Source: CAD feature listing. Evaluate the final solid. Frame: model axes, mm. A direction names the side the tool comes from. Give positions to 0.01 mm unless a question says otherwise; leave off trailing zeros. Loops run counter-clockwise (first coordinate to the right, second up) from the corner with the lowest first, then second, coordinate; pieces in that order, holes last.
from build123d import *
from build123d.topology import SkipClean

# Parameters (mm, degrees)
BOSS_EXTRU_1_DEPTH      = 20
COQUE1_START            = -48.5
COQUE1_OUTLINE_W        = 78
COQUE1_OUTLINE_H        = 18
COQUE1_DEPTH            = 97
ENL_V_MAT_EXTRU_1_DEPTH = 99.357765326
ESQUISSE3_W             = 3
ESQUISSE3_H             = 5
ESQUISSE3_W_2           = 6
ESQUISSE3_H_2           = 3
BOSS_EXTRU_2_DEPTH      = 8
ESQUISSE4_W             = 1.5
ESQUISSE4_H             = 2
ENL_V_MAT_EXTRU_2_DEPTH = 5
CHANFREIN1_SIZE         = 2
ESQUISSE5_W             = 2
ESQUISSE5_H             = 2
ENL_V_MAT_EXTRU_3_DEPTH = 6
CHANFREIN2_SIZE         = 2
ESQUISSE7_W             = 8
ESQUISSE7_H             = 3
ENL_V_MAT_EXTRU_4_DEPTH = 6
CHANFREIN3_SIZE         = 1
ESQUISSE9_R             = 1
ENL_V_MAT_EXTRU_5_DEPTH = 68.492592186
ESQUISSE10_R            = 1
BOSS_EXTRU_5_DEPTH      = 20
ENL_V_MAT_EXTRU_6_DEPTH = 82


# Read off the part's stored shape, not the designer's step: Coque1
with BuildPart() as part:
    # Esquisse1 → Boss.-Extru.1 (new body)
    with BuildSketch(Plane.XY):
        with BuildLine():
            Line((-39, 50.5), (39, 50.5))
            ThreePointArc((39, 50.5), (40.414213562, 49.914213562), (41, 48.5))
            Line((41, 48.5), (41, -48.5))
            ThreePointArc((41, -48.5), (40.414213562, -49.914213562), (39, -50.5))
            Line((39, -50.5), (-39, -50.5))
            ThreePointArc((-39, -50.5), (-40.414213562, -49.914213562), (-41, -48.5))
            Line((-41, -48.5), (-41, 48.5))
            ThreePointArc((-41, 48.5), (-40.414213562, 49.914213562), (-39, 50.5))
        make_face()
    extrude(amount=BOSS_EXTRU_1_DEPTH)

    # Coque1 outline → Coque1 (cut)
    with BuildSketch(Plane(origin=(0, 0, 0), x_dir=(1, 0, 0), z_dir=(0, 1, 0)).offset(COQUE1_START)):
        with Locations((0, -11)):
            Rectangle(COQUE1_OUTLINE_W, COQUE1_OUTLINE_H)
    extrude(amount=COQUE1_DEPTH, mode=Mode.SUBTRACT)

    # Esquisse2 → Enlèv. mat.-Extru.1 (cut, through all)
    with BuildSketch(Plane.ZY.offset(41)):
        Polygon((20, -50.5), (15, -50.5), (20, 50.5), align=None)
    extrude(amount=-ENL_V_MAT_EXTRU_1_DEPTH, mode=Mode.SUBTRACT)

    # Esquisse3 → Boss.-Extru.2 (add)
    with BuildSketch(Plane.XY.offset(2)):
        with Locations((10.5, 40.982596477)):
            Rectangle(ESQUISSE3_W, ESQUISSE3_H)
        with Locations((-10.5, 40.982596477)):
            Rectangle(ESQUISSE3_W, ESQUISSE3_H)
        with Locations((0, 15.010755302)):
            Rectangle(ESQUISSE3_W_2, ESQUISSE3_H_2)
    extrude(amount=BOSS_EXTRU_2_DEPTH)

    # Esquisse4 → Enlèv. mat.-Extru.2 (cut)
    with BuildSketch(Plane.XZ.offset(-38.482596477)):
        with Locations((9.75, 7)):
            Rectangle(ESQUISSE4_W, ESQUISSE4_H)
        with Locations((-9.75, 7)):
            Rectangle(ESQUISSE4_W, ESQUISSE4_H)
    extrude(amount=-ENL_V_MAT_EXTRU_2_DEPTH, mode=Mode.SUBTRACT)

    # Chanfrein1
    chanfrein1_edges = [part.edges().sort_by_distance(p)[0] for p in [
        (9, 40.982596477, 10),
        (-9, 40.982596477, 10),
    ]]
    chamfer(chanfrein1_edges, length=CHANFREIN1_SIZE - 0.0001)  # a hair under: the kernel refuses the full size

    # Esquisse5 → Enlèv. mat.-Extru.3 (cut)
    with BuildSketch(Plane.ZY.offset(3)):
        with Locations((7, 15.510755302)):
            Rectangle(ESQUISSE5_W, ESQUISSE5_H)
    extrude(amount=-ENL_V_MAT_EXTRU_3_DEPTH, mode=Mode.SUBTRACT)

    # Chanfrein2
    chanfrein2_edges = [part.edges().sort_by_distance(p)[0] for p in [
        (0, 16.510755302, 10),
    ]]
    chamfer(chanfrein2_edges, length=CHANFREIN2_SIZE - 0.0001)  # a hair under: the kernel refuses the full size

    # Esquisse7 → Enlèv. mat.-Extru.4 (cut)
    with BuildSketch(Plane(origin=(0, 50.5, 0), x_dir=(1, 0, 0), z_dir=(0, 1, 0))):
        with Locations((0, -8.5)):
            Rectangle(ESQUISSE7_W, ESQUISSE7_H)
    extrude(amount=-ENL_V_MAT_EXTRU_4_DEPTH, mode=Mode.SUBTRACT)

    # Chanfrein3
    chanfrein3_edges = [part.edges().sort_by_distance(p)[0] for p in [
        (4, 49.5, 7),
        (-4, 49.5, 7),
    ]]
    chamfer(chanfrein3_edges, length=CHANFREIN3_SIZE)

    # Esquisse9 → Enlèv. mat.-Extru.5 (cut, through all)
    with BuildSketch(Plane.XY.offset(2)):
        with Locations((-39, 48.5)):
            Circle(ESQUISSE9_R)
        with Locations((-39, -48.5)):
            Circle(ESQUISSE9_R)
        with Locations((-39, 0)):
            Circle(ESQUISSE9_R)
        with Locations((39, 0)):
            Circle(ESQUISSE9_R)
        with Locations((39, -48.5)):
            Circle(ESQUISSE9_R)
        with Locations((39, 48.5)):
            Circle(ESQUISSE9_R)
    extrude(amount=ENL_V_MAT_EXTRU_5_DEPTH, mode=Mode.SUBTRACT)

    # Esquisse10 → Boss.-Extru.5 (add)
    # profile 1 of 12: a face of its own
    with SkipClean():  # the faces are left unmerged after this step: merging them gives an invalid solid
        with BuildSketch(Plane.XY):
            with BuildLine():
                Line((-41, 48.5), (-41, 47))
                ThreePointArc((-41, 47), (-38.209430585, 46.128291755), (-36.5, 48.5))
                ThreePointArc((-36.5, 48.5), (-36.763932023, 49.618033989), (-37.5, 50.5))
                Line((-37.5, 50.5), (-39, 50.5))
                ThreePointArc((-39, 50.5), (-40.414213562, 49.914213562), (-41, 48.5))
            make_face()
            with Locations((-39, 48.5)):
                Circle(ESQUISSE10_R, mode=Mode.SUBTRACT)
        # profile 2 of 12: a face of its own
        with BuildSketch(Plane.XY):
            with BuildLine():
                Line((39, 50.5), (37.5, 50.5))
                ThreePointArc((37.5, 50.5), (37.232233047, 46.732233047), (41, 47))
                Line((41, 47), (41, 48.5))
                ThreePointArc((41, 48.5), (40.414213562, 49.914213562), (39, 50.5))
            make_face()
            with Locations(Location((39, 48.5, 0), (0, 0, 180))):
                Circle(ESQUISSE10_R, mode=Mode.SUBTRACT)
        # profile 3 of 12: a face of its own
        with BuildSketch(Plane.XY):
            with BuildLine():
                ThreePointArc((-40, 0), (-39, 1), (-38, 0))
                Line((-38, 0), (-36.5, 0))
                ThreePointArc((-36.5, 0), (-38.209430585, 2.371708245), (-41, 1.5))
                Line((-41, 1.5), (-41, 0))
                Line((-41, 0), (-40, 0))
            make_face()
        # profile 4 of 12: a face of its own
        with BuildSketch(Plane.XY):
            with BuildLine():
                Line((-36.5, 0), (-38, 0))
                ThreePointArc((-38, 0), (-39, -1), (-40, 0))
                Line((-40, 0), (-41, 0))
                Line((-41, 0), (-41, -1.5))
                ThreePointArc((-41, -1.5), (-38.209430585, -2.371708245), (-36.5, 0))
            make_face()
        # profile 5 of 12: a face of its own
        with BuildSketch(Plane.XY):
            with BuildLine():
                ThreePointArc((-40, 0), (-39, 1), (-38, 0))
                Line((-38, 0), (-36.5, 0))
                ThreePointArc((-36.5, 0), (-38.209430585, 2.371708245), (-41, 1.5))
                Line((-41, 1.5), (-41, 0))
                Line((-41, 0), (-40, 0))
            make_face()
        # profile 6 of 12: a face of its own
        with BuildSketch(Plane.XY):
            with BuildLine():
                Line((-36.5, 0), (-38, 0))
                ThreePointArc((-38, 0), (-39, -1), (-40, 0))
                Line((-40, 0), (-41, 0))
                Line((-41, 0), (-41, -1.5))
                ThreePointArc((-41, -1.5), (-38.209430585, -2.371708245), (-36.5, 0))
            make_face()
        # profile 7 of 12: a face of its own
        with BuildSketch(Plane.XY):
            with BuildLine():
                ThreePointArc((-36.5, -48.5), (-38.209430585, -46.128291755), (-41, -47))
                Line((-41, -47), (-41, -48.5))
                ThreePointArc((-41, -48.5), (-40.414213562, -49.914213562), (-39, -50.5))
                Line((-39, -50.5), (-37.5, -50.5))
                ThreePointArc((-37.5, -50.5), (-36.763932023, -49.618033989), (-36.5, -48.5))
            make_face()
            with Locations(Location((-39, -48.5, 0), (0, 0, 180))):
                Circle(ESQUISSE10_R, mode=Mode.SUBTRACT)
        # profile 8 of 12: a face of its own
        with BuildSketch(Plane.XY):
            with BuildLine():
                ThreePointArc((41, -47), (37.232233047, -46.732233047), (37.5, -50.5))
                Line((37.5, -50.5), (39, -50.5))
                ThreePointArc((39, -50.5), (40.414213562, -49.914213562), (41, -48.5))
                Line((41, -48.5), (41, -47))
            make_face()
            with Locations((39, -48.5)):
                Circle(ESQUISSE10_R, mode=Mode.SUBTRACT)
        # profile 9 of 12: a face of its own
        with BuildSketch(Plane.XY):
            with BuildLine():
                ThreePointArc((41, 1.5), (38.209430585, 2.371708245), (36.5, 0))
                Line((36.5, 0), (38, 0))
                ThreePointArc((38, 0), (39, 1), (40, 0))
                Line((40, 0), (41, 0))
                Line((41, 0), (41, 1.5))
            make_face()
        # profile 10 of 12: a face of its own
        with BuildSketch(Plane.XY):
            with BuildLine():
                Line((38, 0), (36.5, 0))
                ThreePointArc((36.5, 0), (38.209430585, -2.371708245), (41, -1.5))
                Line((41, -1.5), (41, 0))
                Line((41, 0), (40, 0))
                ThreePointArc((40, 0), (39, -1), (38, 0))
            make_face()
        # profile 11 of 12: a face of its own
        with BuildSketch(Plane.XY):
            with BuildLine():
                ThreePointArc((41, 1.5), (38.209430585, 2.371708245), (36.5, 0))
                Line((36.5, 0), (38, 0))
                ThreePointArc((38, 0), (39, 1), (40, 0))
                Line((40, 0), (41, 0))
                Line((41, 0), (41, 1.5))
            make_face()
        # profile 12 of 12: a face of its own
        with BuildSketch(Plane.XY):
            with BuildLine():
                Line((38, 0), (36.5, 0))
                ThreePointArc((36.5, 0), (38.209430585, -2.371708245), (41, -1.5))
                Line((41, -1.5), (41, 0))
                Line((41, 0), (40, 0))
                ThreePointArc((40, 0), (39, -1), (38, 0))
            make_face()
        extrude(amount=BOSS_EXTRU_5_DEPTH)
    add(part.part.scale(1), mode=Mode.REPLACE)  # the faces are merged on a copy

    # Esquisse11 → Enlèv. mat.-Extru.6 (cut)
    with BuildSketch(Plane(origin=(-41, 0, -41), x_dir=(0, 0, 1), z_dir=(-1, 0, 0))):
        Polygon((61, -50.68921089), (56, -50.68921089), (61, 50.5), align=None)
    extrude(amount=-ENL_V_MAT_EXTRU_6_DEPTH, mode=Mode.SUBTRACT)


solid = part.part
1) Contact query for flat-ended pins moving along their axis: P1, Ø2.5, axis at x = 39, y = -48.5, coming from the +Z side; P2, Ø2.5, axis at x = -39, y = 0, coming from the +Z side; P3, Ø1, axis at x = 5, y = 2, coming from the +Z side. Output: stop coordinate, or through.
Checks:
P1: stops at z = 15.17
P2: stops at z = 17.57
P3: stops at z = 2
2) Pull-direction query (Y, two-part tool) for faces 1 (the flat face through (1, -50.5, 7)), 2 (the cylindrical face through (-40.43, 49.9, 9.86)), 3 (the flat face through (-4, 50, 9)), 4 (the flat face through (0, 16.511, 4)); classes: released by +Y, released by -Y, zero draft, split by the parting line, or undercut.
Checks:
face 1: released by -Y
face 2: released by +Y
face 3: zero draft
face 4: undercut
3) Ray query, probe 1 along X at (y, z) = (11, 16); probe 2 along Y at (x, z) = (9.5, 2.5); probe 3 along Y at (x, z) = (35.5, 14.75). Return the intervals inside material, ascending.
Checks:
probe 1: x = -41 to -39, 39 to 41
probe 2: y = -50.5 to -48.5, 38.48 to 43.48, 48.5 to 50.5
probe 3: y = -50.5 to -48.5, 48.5 to 50.5
4) Reachability of faces 5 (the flat face through (38.72, -47.28, 15.17)), 6 (the flat face through (0, 50, 7)), 7 (the flat face through (12, 41, 6)) from +Z, -Z, +X, -X, +Y, -Y: full face, straight path, thin tool, end or side. Return the list, or none.
Checks:
face 5: +Z, +X, -X, -Y
face 6: +Y
face 7: +Z
5) Cut plane B-B (x = 25). Return loops of the section in (y, z).
Checks:
outline: (-50.5, 0) - (50.5, 0) - (50.5, 20) - (48.5, 19.9) - (48.5, 2) - (-48.5, 2) - (-48.5, 15.1) - (-50.5, 15) - close
6) Cut plane A-A (z = 12.5). Return loops of the section in (x, y), and give its area (3 significant figures).
Checks:
outline: (-41, -48.5) arc R2 ccw to (-39, -50.5) - (39, -50.5) arc R2 ccw to (41, -48.5) - (41, 48.5) arc R2 ccw to (39, 50.5) - (-39, 50.5) arc R2 ccw to (-41, 48.5) - close; hole circle Ø2 at (-39, -48.5); hole circle Ø2 at (-39, 0); hole circle Ø2 at (-39, 48.5); hole (-39, -46) arc R2.5 cw to (-36.5, -48.5) - (36.5, -48.5) arc R2.5 cw to (39, -46) - (39, -2.5) arc R2.5 cw to (39, 2.5) - (39, 46) arc R2.5 cw to (36.5, 48.5) - (-36.5, 48.5) arc R2.5 cw to (-39, 46) - (-39, 2.5) arc R2.5 cw to (-39, -2.5) - close; hole circle Ø2 at (39, -48.5); hole circle Ø2 at (39, 0); hole circle Ø2 at (39, 48.5)
area: 733 mm2
7) Cut plane C-C (y = -18.5). Return loops of the section in (x, z).
Checks:
outline: (-41, 0) - (41, 0) - (41, 16.58) - (39, 16.58) - (39, 2) - (-39, 2) - (-39, 16.58) - (-41, 16.58) - close
